```python
from build123d import *

# Parameters (mm, degrees)
F0_R          = 24.5
F1_DEPTH      = 70
F1_DEPTH_BACK = 30
F2_R          = 22.5
F3_DEPTH      = 81.3
F4_R          = 12
F5_DEPTH      = 41.2
F6_R          = 5
F7_SIZE2      = 2.0952461695
F7_SIZE       = 60


# Not quite as in the source:
# - a fillet or chamfer that OpenCascade refuses, or shapes differently, is made with other operations: its cross-section is extruded or revolved along the edge and cut away or added


with BuildPart() as f1:
    # F0 (on Top) → F1 (new body, two sides)
    with BuildSketch(Plane.XY) as f1_sk:
        Circle(F0_R)
    extrude(amount=F1_DEPTH)
    extrude(f1_sk.sketch, amount=-F1_DEPTH_BACK)

    # F2 (on Top) → F3 (cut)
    with BuildSketch(Plane.XY):
        Circle(F2_R)
    extrude(amount=F3_DEPTH, mode=Mode.SUBTRACT)

    # F4 (on Top) → F5 (cut)
    with BuildSketch(Plane.XY):
        Circle(F4_R)
    extrude(amount=-F5_DEPTH, mode=Mode.SUBTRACT)

    # F6
    f6_edges = [f1.edges().sort_by_distance(p)[0] for p in [
        (-12, 0, -30),
    ]]
    fillet(f6_edges, radius=F6_R)

    # F7
    f7_edges = [f1.edges().sort_by_distance(p)[0] for p in [
        (-24.5, 0, -30),
    ]]
    f7_side = f1.faces().sort_by_distance((-24.5, 0, -15))[0]
    chamfer(f7_edges, length=F7_SIZE, length2=F7_SIZE2, reference=f7_side)

    # F8: fillet of radius 5 on 1 edges, made by hand

    # F8_s1 → F8_t2 (revolve, cut)
    with BuildSketch(Plane.XZ):
        with BuildLine():
            ThreePointArc((24.5, 70), (23.027864045, 68.2360679775), (22.5, 66))
            Line((22.5, 66), (22.5, 70))
            Line((22.5, 70), (24.5, 70))
        make_face()
    revolve(axis=Axis((0, 0, 70), (0, 0, -1)), mode=Mode.SUBTRACT)


solid = f1.part
```
Geometry check sheet. Reference: the model listing, model coordinates, mm. Coordinates: 2 decimals unless noted, no trailing zeros. Order: outer loops, then holes, each group sorted by start corner. A loop starts at its lowest first (then second) coordinate and runs counter-clockwise, first axis right, second up. Notation, with made-up numbers: (39, 88) - (78, 88) arc R28 cw to (78, 114) - close; hole circle Ø4 at (84, -21). An arc over 180 degrees is marked (long way). Answer as a JSON object with one key per item and string values. Group by question number.
Item 1: Depth check by flat-ended pin: pin 1 Ø10 at (x, y) = (-10, 1.5) entering from +Z; pin 2 Ø1.5 at (y, z) = (-10, 59) entering from -X; pin 3 Ø10 at (x, z) = (18, 23.5) entering from -Y (3 decimals); pin 4 Ø8 at (x, y) = (-15, -14.5) entering from +Z. Enter the tip coordinate at first touch or a pass-through.
Item 2: Scan lines: probe 1 along X at (y, z) = (1, 30.5); probe 2 along Z at (x, y) = (-4.5, 18); probe 3 along Y at (x, z) = (0, -7.75). Record each from-to range of solid material in increasing order.
Item 3: Sectioned sample at A-A, the plane x = 0. Record the cut outline in (y, z), and give its area (3 significant figures).
Item 4: Sectioned sample at C-C, the plane z = 61.5. Record the cut outline in (x, y).
Item 5: Sectioned sample at D-D, the plane z = 1.5. Record the cut outline in (x, y), and give its area (3 significant figures).
Item 6: Draft check along X on faces 1 (the face through (10, -10, 0)), 2 (the face through (-5.08, -22.88, -0.42)), 3 (the face through (-3, 17, -30)), 4 (the face through (10.382, -19.961, 32.538)). Enter one of: +X half, -X half, draft (parallel to the pull), parting line (faces both ways), or undercut.
Resolved:
{
 "1": {"pin 1": "z = 0", "pin 2": "x = -22.69", "pin 3": "y = -20.505", "pin 4": "z = 70"},
 "2": {"probe 1": "-24.48 to -22.48, 22.48 to 24.48", "probe 2": "-30 to 0", "probe 3": "-23.18 to -12, 12 to 23.18"},
 "3": {"outline": "(-24.5, 30) - (-22.4, -30) - (-17, -30) arc R5 ccw to (-12, -25) - (-12, 0) - (-22.5, 0) - (-22.5, 66) arc R5 ccw to (-24.5, 70) - close; (12, -25) arc R5 ccw to (17, -30) - (22.4, -30) - (24.5, 30) - (24.5, 70) arc R5 ccw to (22.5, 66) - (22.5, 0) - (12, 0) - close", "area": "889 mm^2"},
 "4": {"outline": "circle Ø49 at (0, 0); hole circle Ø45 at (0, 0)"},
 "5": {"outline": "circle Ø47.01 at (0, 0); hole circle Ø45 at (0, 0)", "area": "145 mm^2"},
 "6": {"face 1": "undercut", "face 2": "parting line", "face 3": "draft", "face 4": "undercut"}
}
